Geometry: see drawing. Coordinates: mm, zero at the bounding-box minimum. A direction names the side the tool comes from. Round coordinates to 2 decimals unless told otherwise and drop trailing zeros. Loops run counter-clockwise (first coordinate to the right, second up) from the corner with the lowest first, then second, coordinate; pieces in that order, holes last. Notation, with made-up numbers: (7.25, 42.25) - (55.25, 42.25) arc R22 cw to (55.25, 55.25) - close; hole circle Ø7 at (13.5, -29). An arc over 180 degrees is marked (long way). Return JSON: item names as keys, results as strings. Group by question number.
1. Section C-C on y = 2.25. Return loops of the section in (x, z), and give its area (3 significant figures).
2. Set-up query: the marked faces 1 and 2. Return all of +Z, -Z, +X, -X, +Y, -Y with unobstructed straight access to the full face (end or side cutting, diameter ignored); none if empty.
3. Section A-A on x = 2.75. Return loops of the section in (y, z).
4. Section B-B on z = 33. Return loops of the section in (x, y).
5. Material intervals for probe 1 along Y at (x, z) = (8, 33.5); probe 2 along Z at (x, y) = (18.5, 13.25) (1 decimal); probe 3 along Z at (x, y) = (7.75, 8.25) (1 decimal), sorted ascending.
6. First-contact query: pin 1 Ø10 at (y, z) = (14.5, 15.5) entering from +X; pin 2 Ø1.5 at (x, z) = (15, 26.5) entering from +Y; pin 3 Ø6 at (x, y) = (11.5, 15) entering from -Z; pin 4 Ø12 at (x, z) = (19, 14.5) entering from -Y. Flat tips, straight axial feed; report the tip coordinate or a pass-through.
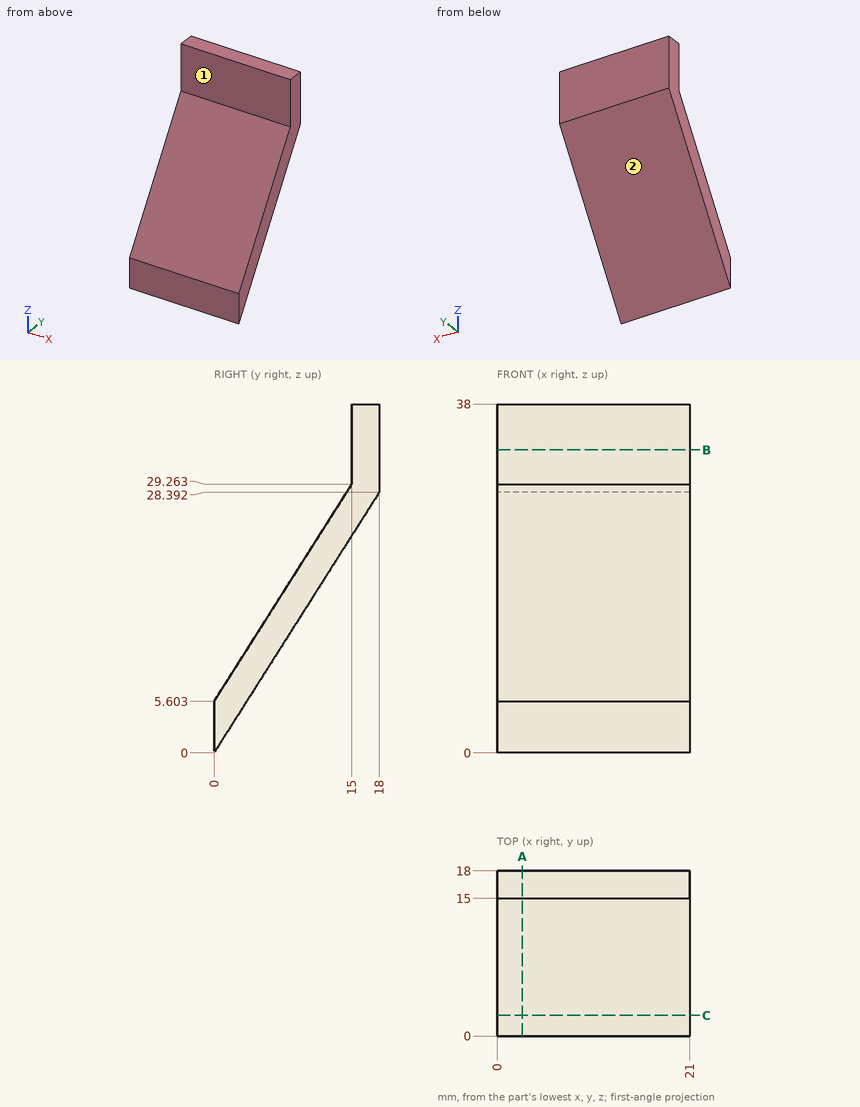
Taken from the geometry:
{
 "1": {"outline": "(0, 3.55) - (21, 3.55) - (21, 9.15) - (0, 9.15) - close", "area": "118 mm2"},
 "2": {"face 1": "+Z, +X, -X, -Y", "face 2": "-Z, +X, -X, +Y"},
 "3": {"outline": "(0, 0) - (18, 28.39) - (18, 38) - (15, 38) - (15, 29.26) - (0, 5.6) - close"},
 "4": {"outline": "(0, 15) - (21, 15) - (21, 18) - (0, 18) - close"},
 "5": {"probe 1": "15 to 18", "probe 2": "20.9 to 26.5", "probe 3": "13 to 18.6"},
 "6": {"pin 1": "x = 21", "pin 2": "y = 17.28", "pin 3": "z = 18.93", "pin 4": "y = 1.84"}
}
